Model file for the job. Use its own axes, mm. A direction names the side the tool comes from. Round coordinates to 2 decimals unless told otherwise and drop trailing zeros. Loops run counter-clockwise (first coordinate to the right, second up) from the corner with the lowest first, then second, coordinate; pieces in that order, holes last. Notation, with made-up numbers: M 68.25,22.25 L 109.25,22.25 A17 ccw 109.25,36.25 Z; hole C 27.25,55 d11. An arc over 180 degrees is marked long. Use a Markdown table: item, result. Add a question column.
Item 1: Wall check: L1, parallel to X at y = 7, z = 7; L2, parallel to Y at x = 6.75, z = 0.75; L3, parallel to X at y = 6, z = 9.25. Give the ranges that are in metal, low to high. Write a range as from..to.
Item 2: Saw through at B-B on z = 7.5. Write the cut outline in (x, y).
Item 3: Saw through at A-A on y = 20. Write the cut outline in (x, z), then the cut area to 3 significant figures.
Item 4: Pin check, flat tips, straight feed: P1, Ø2, axis at x = 7.5, y = 12, coming from the +Z side; P2, Ø3, axis at y = -7.5, z = 7.5, coming from the +X side. Stop position of each tip, or through.
Item 5: Tool access for faces 1 (the cylindrical face through (7.19, 23.71, 3.51)), 2 (the flat face through (7, 4, 3.8)), 3 (the cylindrical face through (7.191, -15.706, 3.499)), 4 (the flat face through (-1, 4, 0)), 5 (the cylindrical face through (-10.38, 4.27, 9.5)): list every direction of +Z, -Z, +X, -X, +Y, -Y with a clear straight run to the whole face (end or side of a thin tool).
```python
from build123d import *

# Parameters (mm, degrees)
F0_W     = 20
F0_H     = 40
F1_DEPTH = 3.8
F2_W     = 17
F2_H     = 40
F3_DEPTH = 6
F4_R     = 1


with BuildPart() as f1:
    # F0 (on Top) → F1 (new body)
    with BuildSketch(Plane.XY):
        with Locations((-0.663412, 4.008531)):
            Rectangle(F0_W, F0_H)
    extrude(amount=F1_DEPTH)

    # F2 (on face) → F3 (join)
    with BuildSketch(Plane.XY.offset(3.8)):
        with Locations((-2.163412, 4.008531)):
            Rectangle(F2_W, F2_H)
    extrude(amount=F3_DEPTH)

    # F4
    f4_edges = [f1.edges().sort_by_distance(p)[0] for p in [
        (6.336588, 4.008531, 9.8),
        (-10.663412, 4.008531, 9.8),
        (9.336588, 4.008531, 3.8),
        (-2.163412, 24.008531, 9.8),
        (9.336588, 24.008531, 1.9),
        (7.836588, 24.008531, 3.8),
        (6.336588, 24.008531, 6.8),
        (-10.663412, 24.008531, 4.9),
        (-0.663412, 24.008531, 0),
        (-10.663412, -15.991469, 4.9),
        (-2.163412, -15.991469, 9.8),
        (6.336588, -15.991469, 6.8),
        (7.836588, -15.991469, 3.8),
        (9.336588, -15.991469, 1.9),
        (-0.663412, -15.991469, 0),
    ]]
    fillet(f4_edges, radius=F4_R)


solid = f1.part
```
Entries:
| question | item | result |
|---|---|---|
| 1 | L1 | -10.66..6.34 |
| 1 | L2 | -15.96..23.98 |
| 1 | L3 | -10.56..6.23 |
| 2 | outline | M -10.66,-14.99 A1 ccw -9.66,-15.99 L 5.34,-15.99 A1 ccw 6.34,-14.99 L 6.34,23.01 A1 ccw 5.34,24.01 L -9.66,24.01 A1 ccw -10.66,23.01 Z |
| 3 | outline | M -10.66,0 L 9.34,0 L 9.34,2.8 A1 ccw 8.34,3.8 L 6.34,3.8 L 6.34,8.8 A1 ccw 5.34,9.8 L -9.66,9.8 A1 ccw -10.66,8.8 Z |
| 3 | area | 177 mm2 |
| 4 | P1 | z = 3.8 |
| 4 | P2 | x = 6.34 |
| 5 | face 1 | +Z, +X, +Y |
| 5 | face 2 | +Z, +X, +Y, -Y |
| 5 | face 3 | +Z, +X, -Y |
| 5 | face 4 | -Z, +X, -X, +Y, -Y |
| 5 | face 5 | +Z, -X, +Y, -Y |
